from build123d import *


with BuildPart() as part:
    # Sketch1 → Revolve1 (revolve)
    with BuildSketch(Plane.XY, mode=Mode.PRIVATE) as revolve1_sk:
        Polygon((0, 0), (0, 25), (40, 25), (40, 40), (60, 40), (60, 25), (80, 25), (80, 20), (100, 20), (100, 15), (120, 15), (120, 10), (140, 10), (140, 5), (160, 5), (160, 0), align=None)
    revolve(revolve1_sk.sketch.rotate(Axis((0, 0, 0), (1, 0, 0)), 90), axis=Axis((0, 0, 0), (1, 0, 0)))  # turned: the seam where the file's is


solid = part.part
Here's how the part is built. I have some questions about the finished solid (model axes, mm). A direction names the side the tool comes from. Coordinates: 2 decimals unless noted, no trailing zeros. Loops run counter-clockwise (first coordinate to the right, second up) from the corner with the lowest first, then second, coordinate; pieces in that order, holes last. Notation, with made-up numbers: (63, 73) -> (120, 73) arc R22 cw to (120, 83) -> close; hole circle Ø1 at (4, -17). An arc over 180 degrees is marked (long way). Use one line per item in the form item = value. Start each with the question number.
(1) Please list where these lines run through material, in increasing order: line 1 along X through (y, z) = (-9.5, -9); line 2 along X through (y, z) = (-8, 33); line 3 along Z through (x, y) = (82, 1).
(2) Will these pins go through, and if not, where does the flat tip stop? pin 1 (1.5 mm diameter, centred on y = -7.5, z = -0.5, fed in from +X); pin 2 (5 mm diameter, centred on x = 103, y = -11, fed in from -Z); pin 3 (2 mm diameter, centred on y = -2.5, z = -29.5, fed in from -X); pin 4 (20 mm diameter, centred on y = -1.5, z = -7.5, fed in from +X).
(3) If we section it at A-A (z = 0): Please give me the cut outline in (x, y).
(4) If we section it at D-D (z = 17): Please give me the cut outline in (x, y).
(5) On a 3-axis mill with a long thin cutter (end or side, diameter ignored), from which of +Z, -Z, +X, -X, +Y, -Y can I reach the whole of each face in a straight line? I mean faces 3 (the face through (0, 0, 0)), 4 (the face through (120, 10, 3)), 5 (the face through (20.28, -7.509, 23.846)). Say none if no direction works.
(6) If we section it at C-C (x = 132.5): Please give me the cut outline in (y, z), then the cut area to 3 significant figures.
(7) We'd pull the mould along Y, two halves only. Please class faces 1 (the face through (150, 0, -5)), 2 (the face through (160, 0, 0)): pulls with the +Y half, pulls with the -Y half, needs draft (parallel to the pull), parting line crosses it, or undercut.
Verdict:
q1.line_1 = 0 to 120
q1.line_2 = 40 to 60
q1.line_3 = -19.97 to 19.97
q2.pin_1 = 140
q2.pin_2 = -12.36
q2.pin_3 = 40
q2.pin_4 = 160
q3.outline = (0, -25) -> (40, -25) -> (40, -40) -> (60, -40) -> (60, -25) -> (80, -25) -> (80, -20) -> (100, -20) -> (100, -15) -> (120, -15) -> (120, -10) -> (140, -10) -> (140, -5) -> (160, -5) -> (160, 5) -> (140, 5) -> (140, 10) -> (120, 10) -> (120, 15) -> (100, 15) -> (100, 20) -> (80, 20) -> (80, 25) -> (60, 25) -> (60, 40) -> (40, 40) -> (40, 25) -> (0, 25) -> close
q4.outline = (0, -18.33) -> (40, -18.33) -> (40, -36.21) -> (60, -36.21) -> (60, -18.33) -> (80, -18.33) -> (80, -10.54) -> (100, -10.54) -> (100, 10.54) -> (80, 10.54) -> (80, 18.33) -> (60, 18.33) -> (60, 36.21) -> (40, 36.21) -> (40, 18.33) -> (0, 18.33) -> close
q5.face_3 = +Z, -Z, -X, +Y, -Y
q5.face_4 = +X
q5.face_5 = -X
q6.outline = circle Ø20 at (0, 0)
q6.area = 314 mm²
q7.face_1 = parting line crosses it
q7.face_2 = needs draft
